Job drawing, mm, ordinate dimensions from the low corner. One solid piece. Coordinates: 2 decimals unless noted, no trailing zeros. Order: outer loops, then holes, each group sorted by start corner. A loop starts at its lowest first (then second) coordinate and runs counter-clockwise, first axis right, second up. Notation, with made-up numbers: (-4, -31.75) - (53, -31.75) arc R32 ccw to (53, 0.25) - close; hole circle Ø9 at (27, 5). An arc over 180 degrees is marked (long way). Use one line per item in the form item = value.
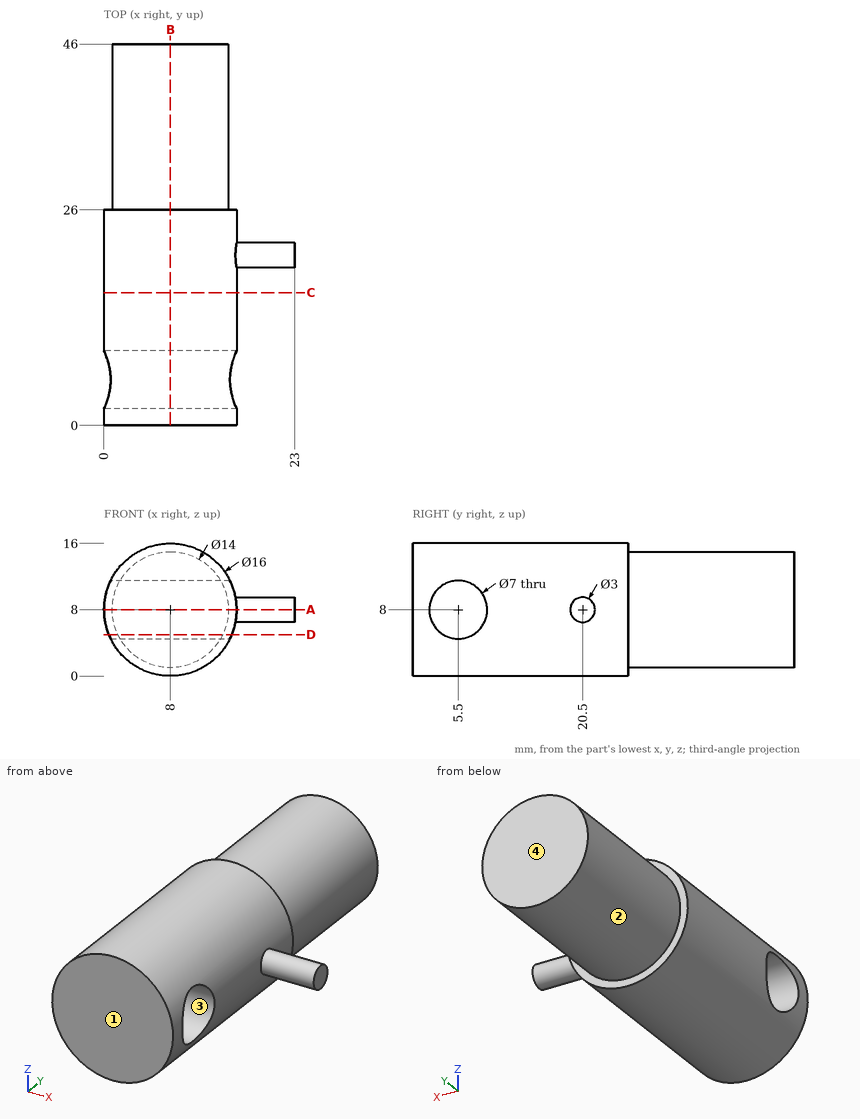
Item 1: Drop flat-ended pins along their axis: pin 1 (5 mm diameter, centred on y = 32, z = 11.5, fed in from +X); pin 2 (12 mm diameter, centred on x = 12.5, y = 34, fed in from +Z); pin 3 (1 mm diameter, centred on y = 13.5, z = 6.5, fed in from +X). Give the stop position or say it passes through.
Derived:
pin_1 = 14.93
pin_2 = 15
pin_3 = 15.94
Item 2: Cut at A-A, the plane z = 8. Write the cut outline in (x, y).
Derived:
outline = (0, 0) - (16, 0) - (16, 2) - (0, 2) - close; (0, 9) - (16, 9) - (16, 19) - (23, 19) - (23, 22) - (16, 22) - (16, 26) - (15, 26) - (15, 46) - (1, 46) - (1, 26) - (0, 26) - close
Item 3: Cut at C-C, the plane y = 16. Write the cut outline in (x, z), plus the area to 3 significant figures.
Derived:
outline = circle Ø16 at (8, 8)
area = 201 mm²
Item 4: Cut at D-D, the plane z = 5. Write the cut outline in (x, y), plus the area to 3 significant figures.
Derived:
outline = (0.58, 0) - (15.42, 0) - (15.42, 3.7) - (0.58, 3.7) - close; (0.58, 7.3) - (15.42, 7.3) - (15.42, 26) - (14.32, 26) - (14.32, 46) - (1.68, 46) - (1.68, 26) - (0.58, 26) - close
area = 585 mm²
Item 5: Cut at B-B, the plane x = 8. Write the cut outline in (y, z), plus the area to 3 significant figures.
Derived:
outline = (0, 0) - (26, 0) - (26, 1) - (46, 1) - (46, 15) - (26, 15) - (26, 16) - (0, 16) - close; hole circle Ø7 at (5.5, 8)
area = 658 mm²
Item 6: Drill centre lines: line 1 (Y direction, x = 4, z = 8); line 2 (Y direction, x = 11.5, z = 9.5); line 3 (Z direction, x = 3, y = 38). Where is each one in solid material? Low to high. Write a range as [from, to].
Derived:
line_1 = [0, 2], [9, 46]
line_2 = [0, 2.34], [8.66, 46]
line_3 = [3.1, 12.9]
Item 7: Two-plate mould, pull along Y, no slides. Class the marked faces 1, 2, 3 and 4: +Y half, -Y half, draft (parallel to the pull), parting line (faces both ways), or undercut.
Derived:
face_1 = -Y half
face_2 = draft
face_3 = undercut
face_4 = +Y half
